Input: dimensioned drawing with shaded views. Units: mm. Origin: part minimum x, y, z. A direction names the side the tool comes from. Round coordinates to 2 decimals unless told otherwise and drop trailing zeros. Write each loop counter-clockwise with the first axis right and the second up, starting at its lowest first coordinate (ties: lowest second). Pieces come first, ordered by that corner, then holes. Notation, with made-up numbers: M 3,68 L 50,68 A20 cw 50,83 Z; hole C 88,47.5 d6. An arc over 180 degrees is marked long. Answer in a Markdown table with one row per item. Add a question column.
Item 1: Cut plane A-A on y = 12.5. Return loops of the section in (x, z).
Item 2: Cut plane D-D on z = 112.5. Return loops of the section in (x, y).
Item 3: Contact query for flat-ended pins moving along their axis: pin 1 (5 mm diameter, centred on x = 16.5, y = 40.5, fed in from -Z); pin 2 (6.5 mm diameter, centred on y = 40.5, z = 137.5, fed in from +X); pin 3 (17.5 mm diameter, centred on x = 19, y = 18.5, fed in from +Z). Output: stop coordinate, or through.
Item 4: Material intervals for probe 1 along Y at (x, z) = (2, 112); probe 2 along Y at (x, z) = (22.5, 2.4); probe 3 along Y at (x, z) = (2.9, 137.5), sorted ascending.
Item 5: Set-up query: the marked faces 1 and 2. Return all of +Z, -Z, +X, -X, +Y, -Y with unobstructed straight access to the full face (end or side cutting, diameter ignored); none if empty.
Item 6: Cut plane B-B on z = 137.5. Return loops of the section in (x, y), and give its area (3 significant figures).
Item 7: Cut plane C-C on x = 22.5. Return loops of the section in (y, z), and give its area (3 significant figures).
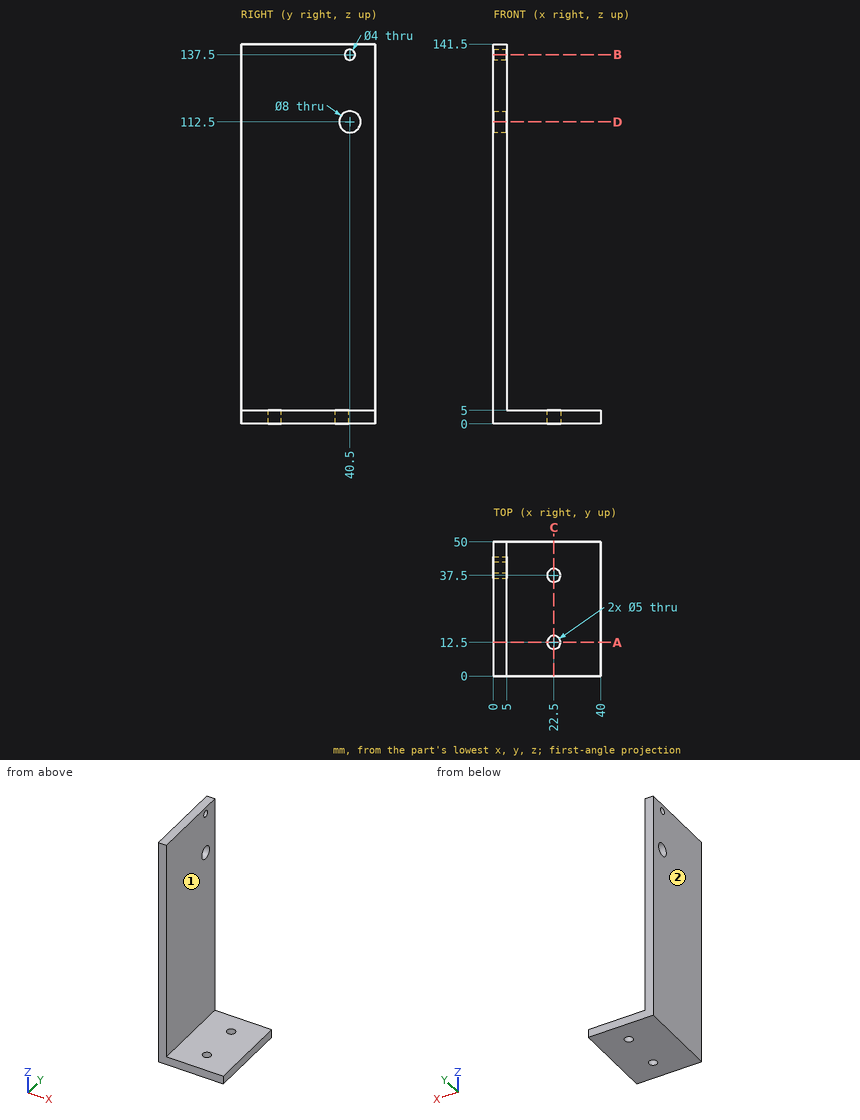
Results below:
| question | item | result |
|---|---|---|
| 1 | outline | M 0,0 L 20,0 L 20,5 L 5,5 L 5,141.5 L 0,141.5 Z; M 25,0 L 40,0 L 40,5 L 25,5 Z |
| 2 | outline | M 0,0 L 5,0 L 5,36.5 L 0,36.5 Z; M 0,44.5 L 5,44.5 L 5,50 L 0,50 Z |
| 3 | pin 1 | z = 0 |
| 3 | pin 2 | x = 5 |
| 3 | pin 3 | z = 5 |
| 4 | probe 1 | 0 to 36.53, 44.47 to 50 |
| 4 | probe 2 | 0 to 10, 15 to 35, 40 to 50 |
| 4 | probe 3 | 0 to 38.5, 42.5 to 50 |
| 5 | face 1 | +Z, +X, +Y, -Y |
| 5 | face 2 | +Z, -Z, -X, +Y, -Y |
| 6 | outline | M 0,0 L 5,0 L 5,38.5 L 0,38.5 Z; M 0,42.5 L 5,42.5 L 5,50 L 0,50 Z |
| 6 | area | 230 mm2 |
| 7 | outline | M 0,0 L 10,0 L 10,5 L 0,5 Z; M 15,0 L 35,0 L 35,5 L 15,5 Z; M 40,0 L 50,0 L 50,5 L 40,5 Z |
| 7 | area | 200 mm2 |
